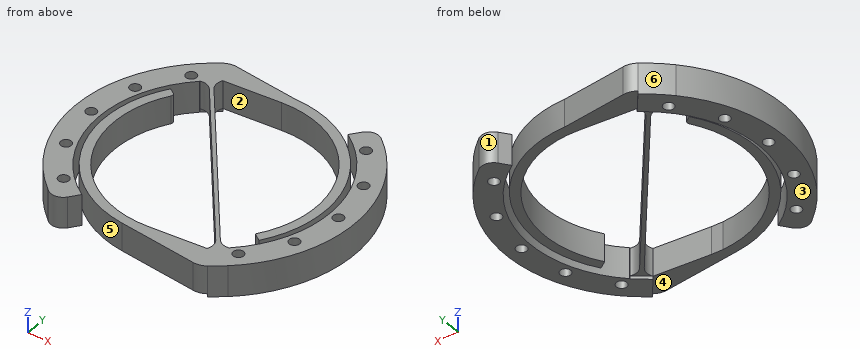
```python
from build123d import *

# Parameters (mm, degrees)
BOSS_EXTRUDE1_DEPTH     = 2.25
BOSS_EXTRUDE2_DEPTH     = 0.5
SKETCH5_R               = 0.850002184
CUT_EXTRUDE1_DEPTH      = 1
CUT_EXTRUDE1_DEPTH_BACK = 6


with BuildPart() as part:
    # Sketch2 → Boss-Extrude1 (new body, symmetric)
    with BuildSketch(Plane.XY):
        with BuildLine():
            Line((2.713147674, 1.38944985), (1.528065997, -0.150989389))
            ThreePointArc((1.528065997, -0.150989389), (0.17725111, -0.917704623), (-1.31492025, -0.486453258))
            Line((-1.31492025, -0.486453258), (-1.753865618, -0.096037363))
            ThreePointArc((-1.753865618, -0.096037363), (-9.620538113, 15.815478855), (-3.478285545, 32.468815395))
            ThreePointArc((-3.478285545, 32.468815395), (-1.657553469, 34.19316142), (0.335322036, 35.715292075))
            ThreePointArc((0.335322036, 35.715292075), (1.310576189, 36.140071747), (2.372755236, 36.197813468))
            Line((2.372755236, 36.197813468), (12.835373957, 34.894529227))
            ThreePointArc((12.835373957, 34.894529227), (28.536577221, 25.247997312), (27.396378685, 6.85551762))
            Line((27.396378685, 6.85551762), (26.165923945, 7.71335154))
            ThreePointArc((26.165923945, 7.71335154), (26.986392928, 24.995972492), (11.764919509, 33.222083557))
            Line((11.764919509, 33.222083557), (2.713147674, 32.624522546))
            ThreePointArc((2.713147674, 32.624522546), (2.470709746, 31.507408509), (2.879736705, 30.439973796))
            Line((2.879736705, 30.439973796), (23.266595715, 3.939876853))
            ThreePointArc((23.266595715, 3.939876853), (24.193426287, 3.270845706), (25.335310798, 3.218717494))
            Line((25.335310798, 3.218717494), (25.335310798, 3.30054722))
            ThreePointArc((25.335310798, 3.30054722), (31.300372108, 18.542612289), (22.957572367, 32.624522546))
            Line((22.957572367, 32.624522546), (24.142654044, 34.164961785))
            ThreePointArc((24.142654044, 34.164961785), (25.492802118, 34.931598224), (26.984595921, 34.501269859))
            ThreePointArc((26.984595921, 34.501269859), (35.334137123, 17.306419127), (27.42640432, -0.096037363))
            Line((27.42640432, -0.096037363), (25.335310798, -1.701329119))
            ThreePointArc((25.335310798, -1.701329119), (24.360060505, -2.126090593), (23.297891975, -2.183826688))
            Line((23.297891975, -2.183826688), (10.641243869, -0.60724147))
            ThreePointArc((10.641243869, -0.60724147), (-3.379346512, 9.784930922), (-1.725632249, 27.158457646))
            Line((-1.725632249, 27.158457646), (-0.899188364, 26.582287247))
            ThreePointArc((-0.899188364, 26.582287247), (-0.694395528, 26.267887803), (-0.765964702, 25.899560545))
            ThreePointArc((-0.765964702, 25.899560545), (-1.606558349, 9.608289856), (12.106530022, 0.772945738))
            Line((12.106530022, 0.772945738), (13.905800532, 0.791888839))
            Line((13.905800532, 0.791888839), (22.957572367, 1.38944985))
            ThreePointArc((22.957572367, 1.38944985), (23.200013724, 2.506566373), (22.790986515, 3.574004371))
            Line((22.790986515, 3.574004371), (2.404127505, 30.074101314))
            ThreePointArc((2.404127505, 30.074101314), (1.477253865, 30.743151427), (0.335322036, 30.795252278))
            Line((0.335322036, 30.795252278), (0.335322036, 30.713422552))
            ThreePointArc((0.335322036, 30.713422552), (-5.629385297, 15.471362635), (2.713147674, 1.38944985))
        make_face()
    extrude(amount=BOSS_EXTRUDE1_DEPTH, both=True)

    # Sketch3 → Boss-Extrude2 (add)
    with BuildSketch(Plane(origin=(0, 0, -2.25), x_dir=(-1, 0, 0), z_dir=(0, 0, -1))):
        with BuildLine():
            Line((-25.335310798, 3.218717494), (-22.957572367, 1.38944985))
            Line((-22.957572367, 1.38944985), (-25.335310798, -1.701329119))
            Line((-25.335310798, -1.701329119), (-27.42640432, -0.096037363))
            ThreePointArc((-27.42640432, -0.096037363), (-35.334137123, 17.306419127), (-26.984595921, 34.501269859))
            ThreePointArc((-26.984595921, 34.501269859), (-25.492802118, 34.931598224), (-24.142654044, 34.164961785))
            Line((-24.142654044, 34.164961785), (-22.957572367, 32.624522546))
            ThreePointArc((-22.957572367, 32.624522546), (-31.300372108, 18.542612289), (-25.335310798, 3.30054722))
            Line((-25.335310798, 3.30054722), (-25.335310798, 3.218717494))
        make_face()
        with BuildLine():
            Line((-0.335322036, 30.795252278), (-2.713147674, 32.624522546))
            Line((-2.713147674, 32.624522546), (-0.335322036, 35.715292075))
            ThreePointArc((-0.335322036, 35.715292075), (1.657553469, 34.19316142), (3.478285545, 32.468815395))
            ThreePointArc((3.478285545, 32.468815395), (9.620538113, 15.815478855), (1.753865618, -0.096037363))
            Line((1.753865618, -0.096037363), (1.31492025, -0.486453258))
            ThreePointArc((1.31492025, -0.486453258), (-0.17725111, -0.917704623), (-1.528065997, -0.150989389))
            Line((-1.528065997, -0.150989389), (-2.713147674, 1.38944985))
            ThreePointArc((-2.713147674, 1.38944985), (5.629385297, 15.471362635), (-0.335322036, 30.713422552))
            Line((-0.335322036, 30.713422552), (-0.335322036, 30.795252278))
        make_face()
    extrude(amount=BOSS_EXTRUDE2_DEPTH)

    # Sketch5 → Cut-Extrude1 (cut, two sides)
    with BuildSketch(Plane(origin=(0, 0, -2.75), x_dir=(-1, 0, 0), z_dir=(0, 0, -1))) as cut_extrude1_sk:
        with Locations((-31.312900109, 24.660626427)):
            Circle(SKETCH5_R)
        with Locations((-32.835321764, 17.006965176)):
            Circle(SKETCH5_R)
        with Locations((-31.312900109, 9.353290058)):
            Circle(SKETCH5_R)
        with Locations((-26.977454917, 2.864826813)):
            Circle(SKETCH5_R)
        with Locations((1.306812691, 2.864826813)):
            Circle(SKETCH5_R)
        with Locations((5.642277886, 24.660626427)):
            Circle(SKETCH5_R)
        with Locations((1.306812691, 31.14910354)):
            Circle(SKETCH5_R)
        with Locations((-26.977454917, 31.14910354)):
            Circle(SKETCH5_R)
        with Locations((5.642277886, 9.353290058)):
            Circle(SKETCH5_R)
        with Locations((7.164679538, 17.006965176)):
            Circle(SKETCH5_R)
    extrude(amount=CUT_EXTRUDE1_DEPTH, mode=Mode.SUBTRACT)
    extrude(cut_extrude1_sk.sketch, amount=-CUT_EXTRUDE1_DEPTH_BACK, mode=Mode.SUBTRACT)


solid = part.part
```
The listing builds one solid part. Answer for the finished solid, in the listing's coordinates (mm). Face numbers are marked on the shaded views. A direction names the side the tool comes from. Coordinates: 2 decimals unless noted, no trailing zeros. Loops run counter-clockwise (first coordinate to the right, second up) from the corner with the lowest first, then second, coordinate; pieces in that order, holes last. Notation, with made-up numbers: (17.5, 65) - (69.5, 65) arc R16 cw to (69.5, 93) - close; hole circle Ø3 at (-31, -8.5). An arc over 180 degrees is marked (long way). Use a Markdown table: item, result. Add a question column.
1) Find the intervals of material crossed by line 1 (X direction, y = 21, z = 1.6); line 2 (Y direction, x = 13.5, z = 1.05); line 3 (Y direction, x = 18.5, z = 0.1), in increasing order.
2) The part is cut by section D-D, the plane y = 28. Give the vertices of the cut face in (x, z).
3) The part is cut by section B-B, the plane y = 20.5. Give the vertices of the cut face in (x, z), and give its area (3 significant figures).
4) The part is cut by section C-C, the plane x = 28.5. Give the vertices of the cut face in (y, z), and give its area (3 significant figures).
5) The part is cut by section A-A, the plane x = 17.5. Give the vertices of the cut face in (y, z), and give its area (3 significant figures).
6) The mould has two halves that part along Y. Classify the marked faces 1, 2 and 3: released by +Y, released by -Y, zero draft, split by the parting line, or undercut.
7) Given pin 1 (6 mm diameter, centred on x = 21, y = 11.5, fed in from -Z); pin 2 (1 mm diameter, centred on x = -5.64, y = 24.66, fed in from -Z); pin 3 (1.5 mm diameter, centred on x = 30, z = -0.5, fed in from -Y); pin 4 (1 mm diameter, centred on x = 28, z = 0, fed in from -Y), each flat-ended and moving along its own axis, determine where each tip first touches the part or whether it passes through.
8) For the marked faces 4, 5 and 6, determine the directions among +Z, -Z, +X, -X, +Y, -Y from which every point of the face is accessible in a straight line to the end or side of a thin tool.
Here are the results:
| question | item | result |
|---|---|---|
| 1 | line 1 | x = -9.29 to -5.25, -4.46 to -2.9, 9.38 to 10.14, 28.59 to 30.1, 30.94 to 34.98 |
| 1 | line 2 | y = -0.96 to 0.79, 15.65 to 16.64, 33.24 to 34.88 |
| 1 | line 3 | y = -1.59 to 1.1, 9.15 to 10.14, 32.24 to 33.91 |
| 2 | outline | (-6.78, -2.75) - (-2.09, -2.75) - (-2.09, 2.25) - (-6.78, 2.25) - close; (4, -2.25) - (4.76, -2.25) - (4.76, 2.25) - (4, 2.25) - close; (24.8, -2.25) - (26.77, -2.25) - (26.77, 2.25) - (24.8, 2.25) - close; (27.8, -2.75) - (32.47, -2.75) - (32.47, 2.25) - (27.8, 2.25) - close |
| 3 | outline | (-9.38, -2.75) - (-5.36, -2.75) - (-5.36, 2.25) - (-9.38, 2.25) - close; (-4.57, -2.25) - (-3.02, -2.25) - (-3.02, 2.25) - (-4.57, 2.25) - close; (9.77, -2.25) - (10.53, -2.25) - (10.53, 2.25) - (9.77, 2.25) - close; (28.71, -2.25) - (30.2, -2.25) - (30.2, 2.25) - (28.71, 2.25) - close; (31.04, -2.75) - (35.06, -2.75) - (35.06, 2.25) - (31.04, 2.25) - close |
| 3 | area | 57.4 mm^2 |
| 4 | outline | (0.88, -2.75) - (7.1, -2.75) - (7.1, 2.25) - (0.88, 2.25) - close; (8.68, -2.25) - (12.68, -2.25) - (12.68, 2.25) - (8.68, 2.25) - close; (21.33, -2.25) - (25.32, -2.25) - (25.32, 2.25) - (21.33, 2.25) - close; (26.96, -2.75) - (33.16, -2.75) - (33.16, 2.25) - (26.96, 2.25) - close |
| 4 | area | 98.0 mm^2 |
| 5 | outline | (-1.46, -2.25) - (1.03, -2.25) - (1.03, 2.25) - (-1.46, 2.25) - close; (10.45, -2.25) - (11.44, -2.25) - (11.44, 2.25) - (10.45, 2.25) - close; (32.57, -2.25) - (34.23, -2.25) - (34.23, 2.25) - (32.57, 2.25) - close |
| 5 | area | 23.1 mm^2 |
| 6 | face 1 | released by +Y |
| 6 | face 2 | undercut |
| 6 | face 3 | zero draft |
| 7 | pin 1 | stops at z = -2.25 |
| 7 | pin 2 | passes through |
| 7 | pin 3 | stops at y = 1.64 |
| 7 | pin 4 | stops at y = -0.03 |
| 8 | face 4 | -Z |
| 8 | face 5 | +Z, -Z |
| 8 | face 6 | +Z, -Z, -X, +Y |
